Geometry check sheet. Reference: the model listing, model coordinates, mm. A direction names the side the tool comes from. Coordinates: 2 decimals unless noted, no trailing zeros. Order: outer loops, then holes, each group sorted by start corner. A loop starts at its lowest first (then second) coordinate and runs counter-clockwise, first axis right, second up. Notation, with made-up numbers: (-20, 89) - (21, 89) arc R15 ccw to (21, 106) - close; hole circle Ø3 at (4, -34). An arc over 180 degrees is marked (long way). Put each result on its own line as item: value.
from build123d import *

# Parameters (mm, degrees)
SKETCH_1_W          = 180
SKETCH_1_H          = 94
EXTRUDE_1_DEPTH     = 3
SKETCH_2_W          = 6
SKETCH_2_H          = 10
EXTRUDE_2_DEPTH     = 8
CHAMFER_2_SIZE      = 6
CHAMFER_1_SIZE      = 6
SKETCH_3_R          = 1.5
CUT_EXTRUDE_1_DEPTH = 204.364205307
SKETCH_4_R          = 1.5
CUT_EXTRUDE_2_DEPTH = 204.224014329
SKETCH_5_W          = 4
SKETCH_5_H          = 47
SKETCH_5_H_2        = 38.5
SKETCH_5_W_2        = 8
SKETCH_5_H_3        = 37
EXTRUDE_3_DEPTH     = 4
CHAMFER_3_SIZE      = 2


with BuildPart() as part:
    # Эскиз1 → Бобышка-Вытянуть1 (new body)
    with BuildSketch(Plane.XY):
        with Locations((90, -47)):
            Rectangle(SKETCH_1_W, SKETCH_1_H)
    extrude(amount=EXTRUDE_1_DEPTH)

    # Эскиз2 → Бобышка-Вытянуть2 (add)
    with BuildSketch(Plane.XY.offset(3)):
        with Locations((3, -89)):
            Rectangle(SKETCH_2_W, SKETCH_2_H)
        with Locations((177, -89)):
            Rectangle(SKETCH_2_W, SKETCH_2_H)
        with Locations((3, -52)):
            Rectangle(SKETCH_2_W, SKETCH_2_H)
        with Locations((177, -52)):
            Rectangle(SKETCH_2_W, SKETCH_2_H)
    extrude(amount=EXTRUDE_2_DEPTH)

    # Фаска2
    chamfer_2_edges = [part.edges().sort_by_distance(p)[0] for p in [
        (3, -57, 3),
        (177, -57, 3),
    ]]
    chamfer(chamfer_2_edges, length=CHAMFER_2_SIZE)

    # Фаска1
    chamfer_1_edges = [part.edges().sort_by_distance(p)[0] for p in [
        (3, -84, 3),
        (177, -84, 3),
    ]]
    chamfer(chamfer_1_edges, length=CHAMFER_1_SIZE)

    # Эскиз3 → Вырез-Вытянуть1 (cut, through all)
    with BuildSketch(Plane(origin=(180, 0, 0), x_dir=(0, 0, -1), z_dir=(1, 0, 0))):
        with Locations((-6, -89)):
            Circle(SKETCH_3_R)
        with Locations((-6, -53)):
            Circle(SKETCH_3_R)
    extrude(amount=-CUT_EXTRUDE_1_DEPTH, mode=Mode.SUBTRACT)

    # Эскиз4 → Вырез-Вытянуть2 (cut, through all)
    with BuildSketch(Plane.XY.offset(3)):
        with Locations((4, -4)):
            Circle(SKETCH_4_R)
        with Locations((176, -4)):
            Circle(SKETCH_4_R)
        with Locations((42, -39)):
            Circle(SKETCH_4_R)
        with Locations((138, -39)):
            Circle(SKETCH_4_R)
    extrude(amount=-CUT_EXTRUDE_2_DEPTH, mode=Mode.SUBTRACT)

    # Эскиз5 → Бобышка-Вытянуть3 (add)
    with BuildSketch(Plane.XY.offset(3)):
        with Locations((42, -70.5)):
            Rectangle(SKETCH_5_W, SKETCH_5_H)
        with Locations((138, -70.5)):
            Rectangle(SKETCH_5_W, SKETCH_5_H)
        with Locations((29, -23.75)):
            Rectangle(SKETCH_5_W, SKETCH_5_H_2)
        with Locations((151, -23.75)):
            Rectangle(SKETCH_5_W, SKETCH_5_H_2)
        with Locations((90, -23)):
            Rectangle(SKETCH_5_W_2, SKETCH_5_H_3)
    extrude(amount=EXTRUDE_3_DEPTH)

    # Фаска3
    # the kernel refuses this chamfer: 2 mm, written as the material it adds along each edge
    with BuildSketch(Plane(origin=(6, -72.856634024, 3), x_dir=(0.9996219169112968, 0, -0.02749587661058627), z_dir=(0, -1, 0))) as chamfer_3_piece_1_section:
        Polygon((CHAMFER_3_SIZE * 0.999621916911, CHAMFER_3_SIZE * 0.0274958766106), (-CHAMFER_3_SIZE * 0.0274958766106, CHAMFER_3_SIZE * 0.999621916911), (0, 0), align=None)
    chamfer_3_piece_1 = extrude(amount=21.143365976, mode=Mode.PRIVATE)
    chamfer_3_piece_1 = split(chamfer_3_piece_1, bisect_by=Plane(origin=(6.672348165, -82.469530213, 7.469530213), z_dir=(0, -0.7071067811865476, -0.7071067811865476)), keep=Keep.TOP, mode=Mode.PRIVATE)
    chamfer_3_piece_1 = chamfer_3_piece_1 - Plane(origin=(6.672348165, -89, 6), x_dir=(0, 0, -1), z_dir=(1, 0, 0)) * Cylinder(1.5, 51, mode=Mode.PRIVATE)
    add(chamfer_3_piece_1)
    with BuildSketch(Plane(origin=(174, -94, 3), x_dir=(-0.9996219169112968, 0, -0.02749587661058639), z_dir=(0, 1, 0))) as chamfer_3_piece_2_section:
        Polygon((CHAMFER_3_SIZE * 0.999621916911, CHAMFER_3_SIZE * 0.0274958766106), (-CHAMFER_3_SIZE * 0.0274958766106, CHAMFER_3_SIZE * 0.999621916911), (0, 0), align=None)
    chamfer_3_piece_2 = extrude(amount=21.143365976, mode=Mode.PRIVATE)
    chamfer_3_piece_2 = split(chamfer_3_piece_2, bisect_by=Plane(origin=(173.327651835, -82.469530213, 7.469530213), z_dir=(0, -0.7071067811865476, -0.7071067811865476)), keep=Keep.TOP, mode=Mode.PRIVATE)
    chamfer_3_piece_2 = chamfer_3_piece_2 - Plane(origin=(173.327651835, -89, 6), x_dir=(0, 0, -1), z_dir=(1, 0, 0)) * Cylinder(1.5, 51, mode=Mode.PRIVATE)
    add(chamfer_3_piece_2)
    with BuildSketch(Plane(origin=(6, -47, 3), x_dir=(0.9996219169112968, 0, -0.02749587661058627), z_dir=(0, -1, 0))) as chamfer_3_piece_3_section:
        Polygon((CHAMFER_3_SIZE * 0.999621916911, CHAMFER_3_SIZE * 0.0274958766106), (-CHAMFER_3_SIZE * 0.0274958766106, CHAMFER_3_SIZE * 0.999621916911), (0, 0), align=None)
    chamfer_3_piece_3 = extrude(amount=21.143365976, mode=Mode.PRIVATE)
    chamfer_3_piece_3 = split(chamfer_3_piece_3, bisect_by=Plane(origin=(6.672348166, -58.527104034, 7.472895966), z_dir=(0, 0.7071067811865476, -0.7071067811865476)), keep=Keep.TOP, mode=Mode.PRIVATE)
    chamfer_3_piece_3 = chamfer_3_piece_3 - Plane(origin=(6.672348166, -53, 6), x_dir=(0, 0, -1), z_dir=(1, 0, 0)) * Cylinder(1.5, 51, mode=Mode.PRIVATE)
    add(chamfer_3_piece_3)
    with BuildSketch(Plane(origin=(174, -68.143365976, 3), x_dir=(-0.9996219169112968, 0, -0.02749587661058639), z_dir=(0, 1, 0))) as chamfer_3_piece_4_section:
        Polygon((CHAMFER_3_SIZE * 0.999621916911, CHAMFER_3_SIZE * 0.0274958766106), (-CHAMFER_3_SIZE * 0.0274958766106, CHAMFER_3_SIZE * 0.999621916911), (0, 0), align=None)
    chamfer_3_piece_4 = extrude(amount=21.143365976, mode=Mode.PRIVATE)
    chamfer_3_piece_4 = split(chamfer_3_piece_4, bisect_by=Plane(origin=(173.327651834, -58.527104034, 7.472895966), z_dir=(0, 0.7071067811865476, -0.7071067811865476)), keep=Keep.TOP, mode=Mode.PRIVATE)
    chamfer_3_piece_4 = chamfer_3_piece_4 - Plane(origin=(173.327651834, -53, 6), x_dir=(0, 0, -1), z_dir=(1, 0, 0)) * Cylinder(1.5, 51, mode=Mode.PRIVATE)
    add(chamfer_3_piece_4)


solid = part.part
Q1. Draft check along X on faces 4 (the flat face through (29, -23, 7)), 5 (the flat face through (90, -41.5, 5)), 6 (the flat face through (0, -48, 3)). Enter one of: pulls with the +X half, pulls with the -X half, needs draft (parallel to the pull), parting line crosses it, or undercut.
Answer block:
face 4: needs draft
face 5: undercut
face 6: pulls with the -X half
Q2. Depth check by flat-ended pin: pin 1 Ø2 at (y, z) = (-76.5, 6) entering from +X; pin 2 Ø2 at (x, z) = (91, 5) entering from +Y; pin 3 Ø1.2 at (y, z) = (-65.5, 5) entering from -X. Enter the tip coordinate at first touch or a pass-through.
Answer block:
pin 1: stops at x = 140
pin 2: stops at y = -4.5
pin 3: stops at x = 40
Q3. Section check B-B on x = 91. Record the boundary of the cut face in (y, z), then the cut area to 3 significant figures.
Answer block:
outline: (-94, 0) - (0, 0) - (0, 3) - (-4.5, 3) - (-4.5, 7) - (-41.5, 7) - (-41.5, 3) - (-94, 3) - close
area: 430 mm^2
Q4. Section check A-A on y = -67. Record the boundary of the cut face in (x, z), then the cut area to 3 significant figures.
Answer block:
outline: (0, 0) - (180, 0) - (180, 3) - (140, 3) - (140, 7) - (136, 7) - (136, 3) - (44, 3) - (44, 7) - (40, 7) - (40, 3) - (0, 3) - close
area: 572 mm^2
Q5. Section check C-C on y = -35.5. Record the boundary of the cut face in (x, z), then the cut area to 3 significant figures.
Answer block:
outline: (0, 0) - (180, 0) - (180, 3) - (153, 3) - (153, 7) - (149, 7) - (149, 3) - (94, 3) - (94, 7) - (86, 7) - (86, 3) - (31, 3) - (31, 7) - (27, 7) - (27, 3) - (0, 3) - close
area: 604 mm^2
Q6. Thickness scan on L1, parallel to X at y = -21.5, z = 5.25; L2, parallel to Z at x = 178, y = -89; L3, parallel to Y at x = 42, z = 1.9. Record the ranges inside material, lowest first. Write a range as [from, to].
Answer block:
L1: x = [27, 31], [86, 94], [149, 153]
L2: z = [0, 4.5], [7.5, 11]
L3: y = [-94, -40.5], [-37.5, 0]
Q7. Access from +Z, -Z, +X, -X, +Y, -Y to the whole of each face (thin tool, end or side, straight path). Record for faces 1 (the flat face through (29, -4.5, 5)), 2 (the flat face through (153, -24, 5)), 3 (the flat face through (42, -70, 7)).
Answer block:
face 1: +Z, +X, -X, +Y
face 2: +Z, +X, +Y, -Y
face 3: +Z, +Y, -Y
Q8. Section check D-D on x = 132.5. Record the boundary of the cut face in (y, z).
Answer block:
outline: (-94, 0) - (0, 0) - (0, 3) - (-94, 3) - close
